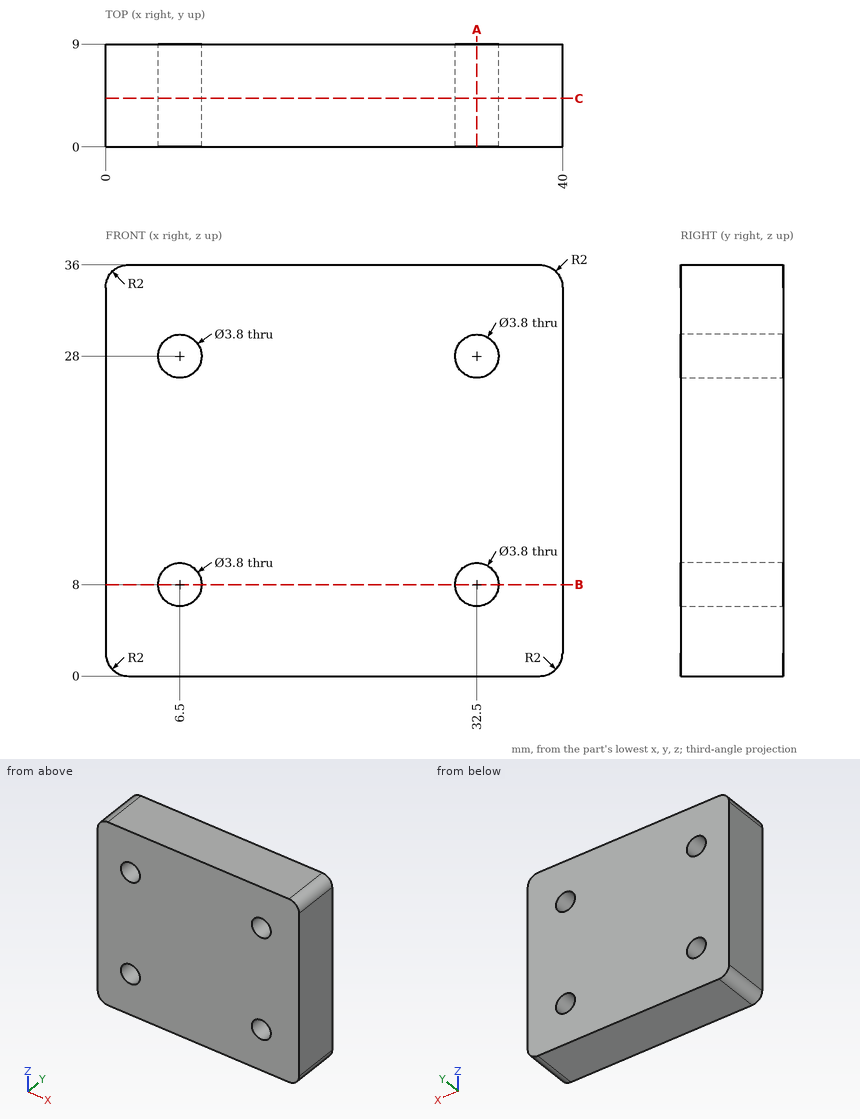
The figure shows three views and two pictorial views of one solid part (mm, origin at its lowest corner). Answer the questions. Round coordinates to 2 decimals unless told otherwise and drop trailing zeros. Order: outer loops, then holes, each group sorted by start corner. A loop starts at its lowest first (then second) coordinate and runs counter-clockwise, first axis right, second up. Notation, with made-up numbers: (49.5, 28) -> (71.5, 28) arc R30 ccw to (71.5, 67) -> close; hole circle Ø11 at (40.5, -2.5). An arc over 180 degrees is marked (long way). Put each result on its own line as item: value.
Q1. Section A-A, the plane x = 32.5 is taken. Write down the section's boundary in (y, z).
Results list:
outline: (0, 0) -> (9, 0) -> (9, 6.1) -> (0, 6.1) -> close; (0, 9.9) -> (9, 9.9) -> (9, 26.1) -> (0, 26.1) -> close; (0, 29.9) -> (9, 29.9) -> (9, 36) -> (0, 36) -> close
Q2. Section B-B, the plane z = 8 is taken. Write down the section's boundary in (x, y).
Results list:
outline: (0, 0) -> (4.6, 0) -> (4.6, 9) -> (0, 9) -> close; (8.4, 0) -> (30.6, 0) -> (30.6, 9) -> (8.4, 9) -> close; (34.4, 0) -> (40, 0) -> (40, 9) -> (34.4, 9) -> close
Q3. Consider line 1 along X through (y, z) = (6.25, 8); line 2 along Z through (x, y) = (32, 1.5); line 3 along Z through (x, y) = (31.5, 2.5). Determine where each line is inside the solid, lowest interval first.
Results list:
line 1: 0 to 4.6, 8.4 to 30.6, 34.4 to 40
line 2: 0 to 6.17, 9.83 to 26.17, 29.83 to 36
line 3: 0 to 6.38, 9.62 to 26.38, 29.62 to 36
Q4. Section C-C, the plane y = 4.25 is taken. Write down the section's boundary in (x, z), and give its area (3 significant figures).
Results list:
outline: (0, 2) arc R2 ccw to (2, 0) -> (38, 0) arc R2 ccw to (40, 2) -> (40, 34) arc R2 ccw to (38, 36) -> (2, 36) arc R2 ccw to (0, 34) -> close; hole circle Ø3.8 at (6.5, 8); hole circle Ø3.8 at (6.5, 28); hole circle Ø3.8 at (32.5, 8); hole circle Ø3.8 at (32.5, 28)
area: 1,390 mm^2
